Here's how the part is built. I have some questions about the finished solid (model axes, mm). Give positions to 0.01 mm unless a question says otherwise; leave off trailing zeros. Loops run counter-clockwise (first coordinate to the right, second up) from the corner with the lowest first, then second, coordinate; pieces in that order, holes last. Notation, with made-up numbers: (78, 84.25) - (123, 84.25) arc R23 ccw to (123, 95.25) - close; hole circle Ø6 at (18.25, -21.75). An arc over 180 degrees is marked (long way). Use a Markdown table: item, result.
from build123d import *

# Parameters (mm, degrees)
BASPROSKE_W         = 3
BASPROSKE_H         = 7
TOOTHCUT_DEPTH      = 11.344080433
TEETHCUTS_COUNT     = 12
HUBNEAONESKE_R      = 2.5
HUBNEARONE_DEPTH    = 8
BORSKE_R            = 0.6
BORE_DEPTH          = 15.0000508
CUT_EXTRUDE_4_DEPTH = 5
SKETCH_2_R          = 3
SKETCH_2_R_2        = 2.5
EXTRUDE_1_DEPTH     = 0.5
SKETCH_3_OUTSIDE_W  = 20.042
SKETCH_3_OUTSIDE_H  = 20.042
SKETCH_3_OUTSIDE_R  = 2.3
CUT_EXTRUDE_5_DEPTH = 5


with BuildPart() as part:
    # BasProSke → Base-Revolve (revolve)
    with BuildSketch(Plane(origin=(0, 0, 0), x_dir=(1, 0, 0), z_dir=(0, 1, 0)), mode=Mode.PRIVATE) as base_revolve_sk:
        with Locations((1.5, 3.5)):
            Rectangle(BASPROSKE_W, BASPROSKE_H)
    revolve(base_revolve_sk.sketch.rotate(Axis((-10, 0, 0), (1, 0, 0)), 180), axis=Axis((-10, 0, 0), (1, 0, 0)))

    # TooCutSke → ToothCut (cut, through all)
    with BuildSketch(Plane(origin=(0, 0, 0), x_dir=(0, 0, -1), z_dir=(1, 0, 0))):
        with BuildLine():
            ThreePointArc((0.562207301, 4.715604304), (0, 4.749), (-0.562207301, 4.715604304))
            ThreePointArc((-0.562207301, 4.715604304), (-0.837528627, 5.917009812), (-1.672850686, 6.823328788))
            ThreePointArc((-1.672850686, 6.823328788), (0, 7.0254), (1.672850686, 6.823328788))
            ThreePointArc((1.672850686, 6.823328788), (0.837528627, 5.917009812), (0.562207301, 4.715604304))
        make_face()
    toothcut = extrude(amount=TOOTHCUT_DEPTH, mode=Mode.SUBTRACT)

    # TeethCuts: ToothCut ×12 about axis
    teethcuts_axis = Axis((0, 0, 0), (1, 0, 0))
    for i in range(1, TEETHCUTS_COUNT):
        add(toothcut.rotate(teethcuts_axis, i * 360 / TEETHCUTS_COUNT), mode=Mode.SUBTRACT)

    # HubNeaOneSke → HubNearOne (add)
    with BuildSketch(Plane.ZY):
        with Locations(Location((0, 0, 0), (0, 0, 180))):
            Circle(HUBNEAONESKE_R)
    extrude(amount=HUBNEARONE_DEPTH)

    # BorSke → Bore (cut, symmetric)
    with BuildSketch(Plane(origin=(0, 0, 0), x_dir=(0, 0, -1), z_dir=(1, 0, 0))):
        with Locations(Location((0, 0, 0), (0, 0, 180))):
            Circle(BORSKE_R)
    extrude(amount=BORE_DEPTH, both=True, mode=Mode.SUBTRACT)

    # 草图1 → 切除-拉伸4 (cut)
    with BuildSketch(Plane.ZY.offset(8)):
        with BuildLine():
            Line((-1.5, 2), (1.5, 2))
            ThreePointArc((1.5, 2), (0, 2.5), (-1.5, 2))
        make_face()
    extrude(amount=-CUT_EXTRUDE_4_DEPTH, mode=Mode.SUBTRACT)

    # 草图2 → 凸台-拉伸1 (add)
    with BuildSketch(Plane.ZY):
        with Locations(Location((0, 0, 0), (0, 0, 180))):
            Circle(SKETCH_2_R)
        with Locations(Location((0, 0, 0), (0, 0, 126.869897646))):
            Circle(SKETCH_2_R_2, mode=Mode.SUBTRACT)
    extrude(amount=EXTRUDE_1_DEPTH)

    # 草图3 outside → 切除-拉伸5 (cut)
    with BuildSketch(Plane.ZY.offset(8)):
        Rectangle(SKETCH_3_OUTSIDE_W, SKETCH_3_OUTSIDE_H)
        Circle(SKETCH_3_OUTSIDE_R, mode=Mode.SUBTRACT)
    extrude(amount=-CUT_EXTRUDE_5_DEPTH, mode=Mode.SUBTRACT)


solid = part.part
(1) Suppose I cut it at D-D on x = -0.25. Write out the boundary of the cut face in (y, z), plus the area to 3 significant figures.
A:
| item | result |
|---|---|
| outline | circle Ø6 at (0, 0); hole circle Ø1.2 at (0, 0) |
| area | 27.1 mm2 |
(2) If I drill on line 1 (Y direction, x = -4.25, z = 0); line 2 (Y direction, x = -2.25, z = 0); line 3 (X direction, y = 2, z = -3), over which ranges is the centre line in solid material (lowest first)?
A:
| item | result |
|---|---|
| line 1 | -2.3 to -0.6, 0.6 to 2 |
| line 2 | -2.5 to -0.6, 0.6 to 2.5 |
| line 3 | 0 to 3 |
(3) Suppose I cut it at C-C on y = 4. Write out the boundary of the cut face in (x, z), plus the area to 3 significant figures.
A:
| item | result |
|---|---|
| outline | (0, -4.87) - (3, -4.87) - (3, -2.96) - (0, -2.96) - close; (0, -2.56) - (3, -2.56) - (3, 2.56) - (0, 2.56) - close; (0, 2.96) - (3, 2.96) - (3, 4.87) - (0, 4.87) - close |
| area | 26.8 mm2 |
(4) Suppose I cut it at B-B on y = 0. Write out the boundary of the cut face in (x, z), plus the area to 3 significant figures.
A:
| item | result |
|---|---|
| outline | (-8, -2.3) - (-3, -2.3) - (-3, -2.5) - (-0.5, -2.5) - (-0.5, -3) - (0, -3) - (0, -4.75) - (3, -4.75) - (3, -0.6) - (-8, -0.6) - close; (-8, 0.6) - (3, 0.6) - (3, 4.75) - (0, 4.75) - (0, 3) - (-0.5, 3) - (-0.5, 2.5) - (-3, 2.5) - (-3, 2.3) - (-8, 2.3) - close |
| area | 53.8 mm2 |
(5) Will these pins go through, and if not, where does the flat tip stop? pin 1 (3 mm diameter, centred on x = -5, y = -3, fed in from -Z); pin 2 (6 mm diameter, centred on x = -2.5, z = 2, fed in from +Y); pin 3 (5 mm diameter, centred on y = -3, z = -4.5, fed in from -X); pin 4 (0.7 mm diameter, centred on x = -5.5, z = 0, fed in from +Y).
A:
| item | result |
|---|---|
| pin 1 | z = -1.74 |
| pin 2 | y = 6.8 |
| pin 3 | x = -0.5 |
| pin 4 | y = 2 |
(6) We'd pull the mould along Z, two halves only. Please class faces 1 (the face through (-6, 2, 0)), 2 (the face through (-1.732, -0.751, -2.385)), 3 (the face through (1.48, 5.51, -2.23)): pulls with the +Z half, pulls with the -Z half, needs draft (parallel to the pull), parting line crosses it, or undercut.
A:
| item | result |
|---|---|
| face 1 | needs draft |
| face 2 | parting line crosses it |
| face 3 | undercut |
(7) Suppose I cut it at A-A on z = 0. Write out the boundary of the cut face in (x, y), plus the area to 3 significant figures.
A:
| item | result |
|---|---|
| outline | (-8, -2.3) - (-3, -2.3) - (-3, -2.5) - (-0.5, -2.5) - (-0.5, -3) - (0, -3) - (0, -4.75) - (3, -4.75) - (3, -0.6) - (-8, -0.6) - close; (-8, 0.6) - (3, 0.6) - (3, 4.75) - (0, 4.75) - (0, 3) - (-0.5, 3) - (-0.5, 2.5) - (-3, 2.5) - (-3, 2) - (-8, 2) - close |
| area | 52.3 mm2 |
